Verification items for this drawing (mm, ordinates from the low corner). A direction names the side the tool comes from. Give positions to 0.01 mm unless a question says otherwise; leave off trailing zeros. Order: outer loops, then holes, each group sorted by start corner. A loop starts at its lowest first (then second) coordinate and runs counter-clockwise, first axis right, second up. Notation, with made-up numbers: M 11,-10 L 22,-10 A34 cw 22,26 Z; hole C 27.5,35.5 d7. An arc over 180 degrees is marked long. Return JSON: item names as keys, results as strings. Group by question number.
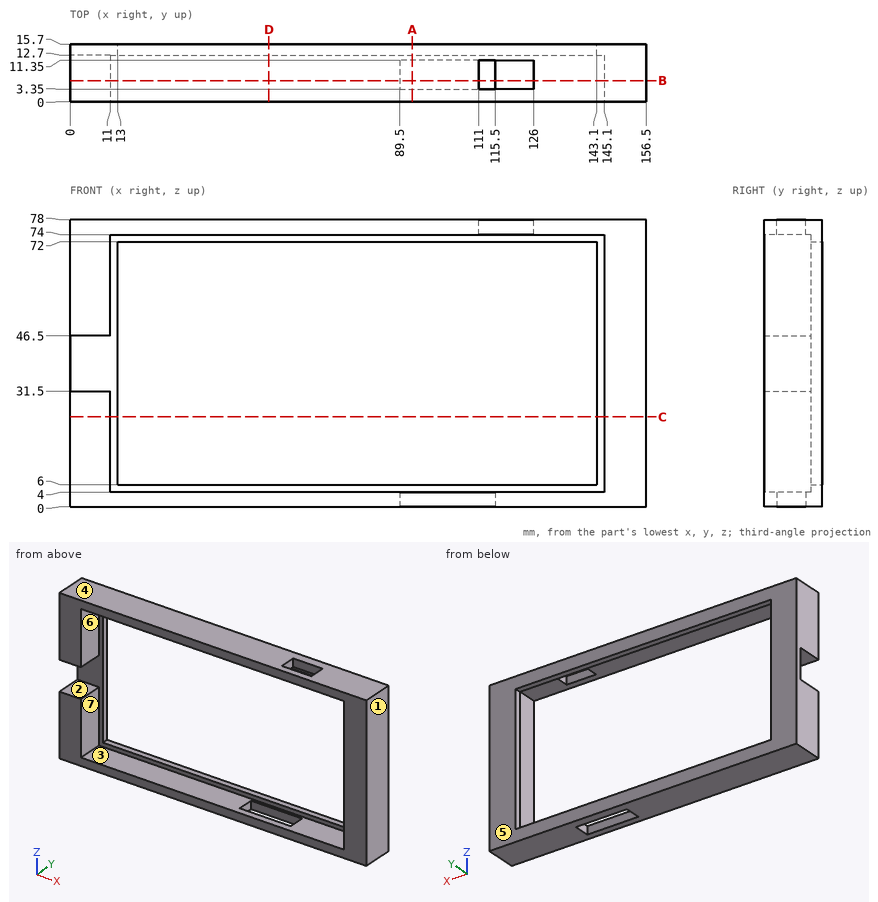
1) Sectioned sample at A-A on x = 93. Record the boundary of the cut face in (y, z).
2) Depth check by flat-ended pin: P1, Ø2, axis at y = 9.5, z = 33, coming from the -X side. Enter the tip coordinate at first touch or a pass-through.
3) Sectioned sample at C-C on z = 24.5. Record the boundary of the cut face in (x, y).
4) Sectioned sample at B-B on y = 5.75. Record the boundary of the cut face in (x, z).
5) Release check for a two-part mould opening along Z. For the marked faces 4, 5, 6 and 7 record: released by +Z, released by -Z, zero draft, split by the parting line, or undercut.
6) Tool access check on the marked faces 1, 2 and 3. Record the directions out of +Z, -Z, +X, -X, +Y, -Y that give a thin tool (end or side, any length) a straight path to the whole face; none if there is none.
7) Material ranges on line 1 along X through (y, z) = (7, 12); line 2 along Z through (x, y) = (142, 11.5); line 3 along X through (y, z) = (14.5, 18.5), recorded low to high.
8) Sectioned sample at D-D on x = 54. Record the boundary of the cut face in (y, z).
Reply:
{
 "1": {"outline": "M 0,0 L 3.35,0 L 3.35,4 L 0,4 Z; M 0,74 L 12.7,74 L 12.7,72 L 15.7,72 L 15.7,78 L 0,78 Z; M 11.35,0 L 15.7,0 L 15.7,6 L 12.7,6 L 12.7,4 L 11.35,4 Z"},
 "2": {"P1": "x = 145.1"},
 "3": {"outline": "M 0,0 L 11,0 L 11,12.7 L 13,12.7 L 13,15.7 L 0,15.7 Z; M 143.1,12.7 L 145.1,12.7 L 145.1,0 L 156.5,0 L 156.5,15.7 L 143.1,15.7 Z"},
 "4": {"outline": "M 0,0 L 89.5,0 L 89.5,4 L 11,4 L 11,31.5 L 0,31.5 Z; M 0,46.5 L 11,46.5 L 11,74 L 111,74 L 111,78 L 0,78 Z; M 115.5,0 L 156.5,0 L 156.5,78 L 126,78 L 126,74 L 145.1,74 L 145.1,4 L 115.5,4 Z"},
 "5": {"face 4": "released by +Z", "face 5": "zero draft", "face 6": "undercut", "face 7": "undercut"},
 "6": {"face 1": "+Z, -Z, +X, +Y, -Y", "face 2": "-X, -Y", "face 3": "-Y"},
 "7": {"line 1": "0 to 11, 145.1 to 156.5", "line 2": "0 to 4, 74 to 78", "line 3": "0 to 13, 143.1 to 156.5"},
 "8": {"outline": "M 0,0 L 15.7,0 L 15.7,6 L 12.7,6 L 12.7,4 L 0,4 Z; M 0,74 L 12.7,74 L 12.7,72 L 15.7,72 L 15.7,78 L 0,78 Z"}
}
